from build123d import *

# Parameters (mm, degrees)
SKETCH_1_W          = 300
SKETCH_1_H          = 36
EXTRUDE_1_DEPTH     = 15
SKETCH_2_R          = 1
CUT_EXTRUDE_2_DEPTH = 5
CUT_EXTRUDE_3_DEPTH = 10
CUT_EXTRUDE_4_REACH = 304.524
SKETCH_5_R          = 1
CUT_EXTRUDE_5_DEPTH = 5
CUT_EXTRUDE_6_REACH = 178.2


with BuildPart() as part:
    # Sketch 1 → Extrude 1 (new body)
    with BuildSketch(Plane.XY):
        with Locations((150, 18)):
            Rectangle(SKETCH_1_W, SKETCH_1_H)
    extrude(amount=EXTRUDE_1_DEPTH)

    # Sketch 2 → Cut-Extrude 2 (cut)
    with BuildSketch(Plane.XY):
        with Locations((9.018599779, 5)):
            Circle(SKETCH_2_R)
        with Locations((7, 18)):
            Circle(SKETCH_2_R)
        with Locations(Location((9.018599779, 31, 0), (0, 0, 180))):
            Circle(SKETCH_2_R)
        with Locations(Location((90.721400221, 5, 0), (0, 0, 180))):
            Circle(SKETCH_2_R)
        with Locations((90.721400221, 31)):
            Circle(SKETCH_2_R)
        with Locations(Location((92.74, 18, 0), (0, 0, 180))):
            Circle(SKETCH_2_R)
    extrude(amount=CUT_EXTRUDE_2_DEPTH, mode=Mode.SUBTRACT)

    # Sketch 3 → Cut-Extrude 3 (cut)
    with BuildSketch(Plane(origin=(0, 0, 0), x_dir=(-1, 0, 0), z_dir=(0, 0, -1))):
        Polygon((-145.169424203, 13), (-145.169424203, 23), (-153.829678241, 28), (-162.489932279, 23), (-162.489932279, 13), (-153.829678241, 8), align=None)
    extrude(amount=-CUT_EXTRUDE_3_DEPTH, mode=Mode.SUBTRACT)

    # Sketch 4 → Cut-Extrude 4 (cut, up to next)
    with BuildSketch(Plane.XY.offset(15), mode=Mode.PRIVATE) as cut_extrude_4_sk1:
        with BuildLine():
            Line((300, 36), (153.829678241, 36))
            ThreePointArc((153.829678241, 36), (171.829678241, 18), (153.829678241, 0))
            Line((153.829678241, 0), (300, 0))
            Line((300, 0), (300, 36))
        make_face()
    cut_extrude_4_tool1 = extrude(cut_extrude_4_sk1.sketch, amount=-CUT_EXTRUDE_4_REACH, mode=Mode.PRIVATE) & part.part
    add(cut_extrude_4_tool1.solids().sort_by_distance((233.9223, 18, 15))[0], mode=Mode.SUBTRACT)

    # Sketch 5 → Cut-Extrude 5 (cut)
    with BuildSketch(Plane(origin=(0, 0, 10), x_dir=(-1, 0, 0), z_dir=(0, 0, -1))):
        with Locations((-153.829678241, 12)):
            Circle(SKETCH_5_R)
        with Locations((-159.829678241, 18)):
            Circle(SKETCH_5_R)
        with Locations((-153.829678241, 24)):
            Circle(SKETCH_5_R)
        with Locations((-147.829678241, 18)):
            Circle(SKETCH_5_R)
    extrude(amount=-CUT_EXTRUDE_5_DEPTH, mode=Mode.SUBTRACT)

    # Sketch 6 → Cut-Extrude 6 (cut, up to next)
    with BuildSketch(Plane(origin=(0, 0, 0), x_dir=(-1, 0, 0), z_dir=(0, 0, -1)), mode=Mode.PRIVATE) as cut_extrude_6_sk1:
        with BuildLine():
            ThreePointArc((0, 18), (-0.847642328, 8.844381598), (-3.361754494, 0))
            Line((-3.361754494, 0), (0, 0))
            Line((0, 0), (0, 18))
        make_face()
    cut_extrude_6_tool1 = extrude(cut_extrude_6_sk1.sketch, amount=-CUT_EXTRUDE_6_REACH, mode=Mode.PRIVATE) & part.part
    # Sketch 6 → Cut-Extrude 6 (cut, up to next)
    with BuildSketch(Plane(origin=(0, 0, 0), x_dir=(-1, 0, 0), z_dir=(0, 0, -1)), mode=Mode.PRIVATE) as cut_extrude_6_sk2:
        with BuildLine():
            ThreePointArc((-3.361754494, 36), (-0.847642328, 27.155618402), (0, 18))
            Line((0, 18), (0, 36))
            Line((0, 36), (-3.361754494, 36))
        make_face()
    cut_extrude_6_tool2 = extrude(cut_extrude_6_sk2.sketch, amount=-CUT_EXTRUDE_6_REACH, mode=Mode.PRIVATE) & part.part
    add(cut_extrude_6_tool1.solids().sort_by_distance((1.002419, 4.469106, 0))[0], mode=Mode.SUBTRACT)
    add(cut_extrude_6_tool2.solids().sort_by_distance((1.002419, 31.530894, 0))[0], mode=Mode.SUBTRACT)


solid = part.part
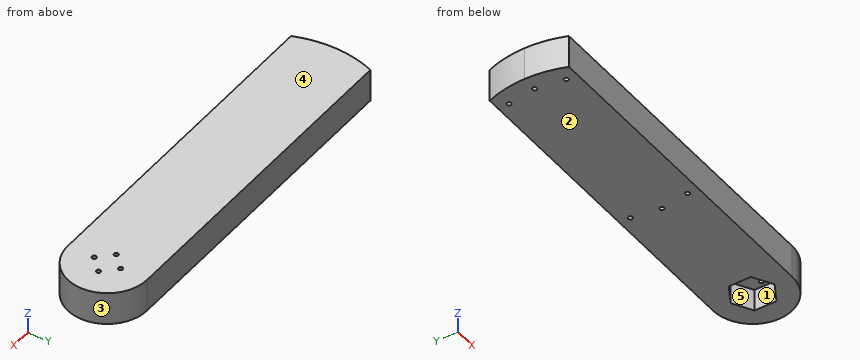
Input: part model. Units: mm. Frame: model coordinates. Face numbers are marked on the shaded views. A direction names the side the tool comes from. Round coordinates to 2 decimals unless told otherwise and drop trailing zeros. Write each loop counter-clockwise with the first axis right and the second up, starting at its lowest first coordinate (ties: lowest second). Pieces come first, ordered by that corner, then holes.
1) Contact query for flat-ended pins moving along their axis: P1, Ø1.8, axis at x = 90.72, y = 31, coming from the -Z side; P2, Ø1.8, axis at x = 159.83, y = 18, coming from the -Z side; P3, Ø2.5, axis at x = 147.83, y = 18, coming from the -Z side; P4, Ø1.5, axis at y = 30.5, z = 11, coming from the -X side. Output: stop coordinate, or through.
2) Cut plane A-A (z = 7). Return the cut outline in (x, y), then the cut area to 3 significant figures.
3) Reachability of the marked faces 4 and 5 from +Z, -Z, +X, -X, +Y, -Y: full face, straight path, thin tool, end or side. Return the list, or none.
4) Ray query, L1, parallel to X at y = 18.5, z = 6; L2, parallel to X at y = 15.5, z = 5.5; L3, parallel to Y at x = 150.5, z = 3. Return the intervals inside material, ascending.
5) Draft query along X for the marked faces 1, 2 and 3. Return one class per face: pulls with the +X half, pulls with the -X half, needs draft (parallel to the pull), parting line crosses it, or undercut.
Geometry says:
1. P1: stops at z = 5
1. P2: passes through
1. P3: stops at z = 10
1. P4: stops at x = 1.4
2. outline: (3.36, 0) - (153.83, 0) arc R18 ccw to (153.83, 36) - (3.36, 36) arc R49.87 ccw to start; hole (145.17, 13) - (153.83, 8) - (162.49, 13) - (162.49, 23) - (153.83, 28) - (145.17, 23) - close
2. area: 5,750 mm2
3. face 4: +Z, +X, -X, +Y, -Y
3. face 5: -Z
4. L1: x = 0 to 145.17, 162.49 to 171.82
4. L2: x = 0.06 to 145.17, 162.49 to 171.66
4. L3: y = 0 to 9.92, 26.08 to 36
5. face 1: undercut
5. face 2: needs draft
5. face 3: pulls with the +X half
